```python
from build123d import *

# Parameters (mm, degrees)
RESSALTO_EXTRUS_O1_DEPTH      = 5
RESSALTO_EXTRUS_O1_DEPTH_BACK = 3
ESBO_O1_R                     = 9
ESBO_O2_R                     = 3
RESSALTO_EXTRUS_O2_DEPTH      = 10
ESBO_O3_R                     = 6
ESBO_O3_R_2                   = 3
CORTE_EXTRUS_O1_DEPTH         = 10


with BuildPart() as part:
    # Esboço1 → Ressalto-extrusão1 (new, two sides: drawn at the far end of the back side and taken through both)
    with BuildSketch(Plane.XY.offset(-RESSALTO_EXTRUS_O1_DEPTH_BACK)):
        Circle(ESBO_O1_R)
    extrude(amount=RESSALTO_EXTRUS_O1_DEPTH + RESSALTO_EXTRUS_O1_DEPTH_BACK)

    # Esboço2 → Ressalto-extrusão2 (add)
    with BuildSketch(Plane.XY):
        Circle(ESBO_O2_R)
    extrude(amount=-RESSALTO_EXTRUS_O2_DEPTH)

    # Esboço3 → Corte-extrusão1 (cut)
    with BuildSketch(Plane.XY):
        Circle(ESBO_O3_R)
        Circle(ESBO_O3_R_2, mode=Mode.SUBTRACT)
    extrude(amount=-CORTE_EXTRUS_O1_DEPTH, mode=Mode.SUBTRACT)


solid = part.part
```
For this review, take the finished solid that the model builds, in its own axes (mm). A direction names the side the tool comes from. Round coordinates to 2 decimals unless told otherwise and drop trailing zeros. Write each loop counter-clockwise with the first axis right and the second up, starting at its lowest first coordinate (ties: lowest second). Pieces come first, ordered by that corner, then holes. Notation, with made-up numbers: (-11.75, -30) -> (10.25, -30) arc R32 cw to (10.25, -3) -> close; hole circle Ø6 at (26, -8.5). An arc over 180 degrees is marked (long way). Use one line per item in the form item = value.
Q1. Machinability: for faces 1 (the flat face through (0, 0, 5)), 2 (the flat face through (-3, -1, 0)), which of the approach directions +Z, -Z, +X, -X, +Y, -Y give a long, thin tool a straight path to every point of the face, cutting with its end or side? Answer none if there is none.
Resolved:
face_1 = +Z, +X, -X, +Y, -Y
face_2 = -Z
Q2. Consider section A-A (y = 0). State the section outline as (x, z) points, then the cut area to 3 significant figures.
Resolved:
outline = (-9, -3) -> (-6, -3) -> (-6, 0) -> (-3, 0) -> (-3, -10) -> (3, -10) -> (3, 0) -> (6, 0) -> (6, -3) -> (9, -3) -> (9, 5) -> (-9, 5) -> close
area = 168 mm²
Q3. Consider section C-C (z = 2.25). State the section outline as (x, y) points.
Resolved:
outline = circle Ø18 at (0, 0)
Q4. The part is to be moulded in two halves that separate along Y. For faces 3 (the cylindrical face through (-1.172, 8.923, 0.944)), 4 (the cylindrical face through (-3, 0, -5)), 5 (the flat face through (2, -6, -3)), 6 (the cylindrical face through (-6, 0, -1)), say which applies: released by +Y, released by -Y, zero draft, split by the parting line, or undercut.
Resolved:
face_3 = split by the parting line
face_4 = undercut
face_5 = zero draft
face_6 = undercut
Q5. To check wall thickness, follow probe 1 along Y at (x, z) = (0, -1.2); probe 2 along X at (y, z) = (-0.25, -1.5); probe 3 along X at (y, z) = (-2.5, -2). State the ranges of each line that lie inside material, in increasing order. Write a range as from..to.
Resolved:
probe_1 = -9..-6, -3..3, 6..9
probe_2 = -9..-5.99, -2.99..2.99, 5.99..9
probe_3 = -8.65..-5.45, -1.66..1.66, 5.45..8.65
Q6. Clearance check with flat-ended pins moving along their axes: pin 1 Ø5 at (x, z) = (-7, -7) entering from +Y; pin 2 Ø8 at (y, z) = (-7, 2.5) entering from -X; pin 3 Ø2 at (y, z) = (5.5, -2) entering from -X; pin 4 Ø6 at (x, y) = (-6, -5.5) entering from -Z. State where each tip first meets the part, or that it passes through.
Resolved:
pin_1 = through
pin_2 = -8.49
pin_3 = -7.79
pin_4 = -3
Q7. Consider section D-D (x = -4.75). State the section outline as (y, z) points, then the cut area to 3 significant figures.
Resolved:
outline = (-7.64, -3) -> (-3.67, -3) -> (-3.67, 0) -> (3.67, 0) -> (3.67, -3) -> (7.64, -3) -> (7.64, 5) -> (-7.64, 5) -> close
area = 100 mm²
